```python
from build123d import *

# Parameters (mm, degrees)
SKETCH1_R            = 41.275
BODY_DEPTH           = 17.78
SKETCH2_R            = 41.275
SKETCH2_R_2          = 32.385
BOTTOM_INITIAL_DEPTH = 12.7
SKETCH3_R            = 32.385
SKETCH3_R_2          = 13.97
BOTTOM_STEM_DEPTH    = 7.62
SKETCH4_W            = 2.286
SKETCH4_H            = 2.54
SKETCH5_W            = 2.286
SKETCH5_H            = 2.54
CHAMFER1_SIZE        = 2.54
CHAMFER1_SIZE2       = 13.97
CUT_EXTRUDE3_REACH   = 63.02
SKETCH9_R            = 2.413
CIRPATTERN1_COUNT    = 6


with BuildPart() as part:
    # Sketch1 → Body (new body)
    with BuildSketch(Plane(origin=(0, 0, 0), x_dir=(1, 0, 0), z_dir=(0, 1, 0))):
        with Locations(Location((0, 0, 0), (0, 0, 270))):
            Circle(SKETCH1_R)
    extrude(amount=BODY_DEPTH)

    # Sketch2 → Bottom Initial (cut)
    with BuildSketch(Plane.XZ):
        with Locations(Location((0, 0, 0), (0, 0, 270))):
            Circle(SKETCH2_R)
        with Locations(Location((0, 0, 0), (0, 0, 270))):
            Circle(SKETCH2_R_2, mode=Mode.SUBTRACT)
    extrude(amount=-BOTTOM_INITIAL_DEPTH, mode=Mode.SUBTRACT)

    # Sketch3 → Bottom Stem (cut)
    with BuildSketch(Plane.XZ):
        with Locations(Location((0, 0, 0), (0, 0, 270))):
            Circle(SKETCH3_R)
        with Locations(Location((0, 0, 0), (0, 0, 270))):
            Circle(SKETCH3_R_2, mode=Mode.SUBTRACT)
    extrude(amount=-BOTTOM_STEM_DEPTH, mode=Mode.SUBTRACT)

    # Sketch4 → Top O ring (revolve, cut)
    with BuildSketch(Plane.XY, mode=Mode.PRIVATE) as top_o_ring_sk:
        with Locations((31.242, 10.16)):
            Rectangle(SKETCH4_W, SKETCH4_H)
    revolve(top_o_ring_sk.sketch.rotate(Axis((0, 18.669, 0), (0, -1, 0)), 270), axis=Axis((0, 18.669, 0), (0, -1, 0)), mode=Mode.SUBTRACT)

    # Sketch5 → Bottom O ring (revolve, cut)
    with BuildSketch(Plane.XY, mode=Mode.PRIVATE) as bottom_o_ring_sk:
        with Locations((12.827, 5.08)):
            Rectangle(SKETCH5_W, SKETCH5_H)
    revolve(bottom_o_ring_sk.sketch.rotate(Axis((0, 18.669, 0), (0, -1, 0)), 270), axis=Axis((0, 18.669, 0), (0, -1, 0)), mode=Mode.SUBTRACT)

    # Chamfer1
    chamfer1_edges = [part.edges().sort_by_distance(p)[0] for p in [
        (0, 0, 13.97),
    ]]
    chamfer1_side = [part.faces().sort_by_distance(p)[0] for p in [
        (0, 1.905, 13.97),
    ]]
    chamfer(chamfer1_edges, length=CHAMFER1_SIZE, length2=CHAMFER1_SIZE2, reference=chamfer1_side[0])

    # Sketch9 → Cut-Extrude3 (cut, up to next)
    with BuildSketch(Plane(origin=(0, 17.78, 0), x_dir=(1, 0, 0), z_dir=(0, 1, 0)), mode=Mode.PRIVATE) as cut_extrude3_sk1:
        with Locations(Location((-36.83, 0, 0), (0, 0, 270))):
            Circle(SKETCH9_R)
    cut_extrude3_tool1 = extrude(cut_extrude3_sk1.sketch, amount=-CUT_EXTRUDE3_REACH, mode=Mode.PRIVATE) & part.part
    cut_extrude3 = cut_extrude3_tool1.solids().sort_by_distance((-36.83, 17.78, 0))[0]
    add(cut_extrude3, mode=Mode.SUBTRACT)

    # CirPattern1: Cut-Extrude3 ×6 about axis
    cirpattern1_axis = Axis((0, 0, 0), (0, 1, 0))
    for i in range(1, CIRPATTERN1_COUNT):
        add(cut_extrude3.rotate(cirpattern1_axis, i * 360 / CIRPATTERN1_COUNT), mode=Mode.SUBTRACT)


solid = part.part
```
The listing builds one solid part. Answer for the finished solid, in the listing's coordinates (mm). A direction names the side the tool comes from. Give positions to 0.01 mm unless a question says otherwise; leave off trailing zeros. Order: outer loops, then holes, each group sorted by start corner. A loop starts at its lowest first (then second) coordinate and runs counter-clockwise, first axis right, second up. Notation, with made-up numbers: (-14, 59) -> (20, 59) arc R17 cw to (20, 84) -> close; hole circle Ø9 at (55.5, 69.5). An arc over 180 degrees is marked (long way). Answer as CSV lines item,"result". Start each with the question number.
Q1. A cutting plane is placed at B-B (y = 14). Determine the outline of the cut face in (x, z) (3 decimals).
Q2. Find the intervals of material crossed by L1, parallel to X at y = 15, z = 0 (3 decimals); L2, parallel to Y at x = 13.5, z = 23.5; L3, parallel to Y at x = 8.5, z = 11, in increasing order.
Q3. Determine the mould class of faces 1 (the cylindrical face through (-18.31, 10.18, 23.89)), 2 (the cylindrical face through (-17.491, 15.276, -34.125)), 3 (the flat face through (-10.3, 6.35, 6.1)) for opening direction X: pulls with the +X half, pulls with the -X half, needs draft (parallel to the pull), parting line crosses it, or undercut.
Q4. Given pin 1 (1.5 mm diameter, centred on x = 2, y = 11.5, fed in from -Z); pin 2 (5.5 mm diameter, centred on x = -18.42, z = 31.9, fed in from -Y); pin 3 (5 mm diameter, centred on y = 11.5, z = 5, fed in from -X); pin 4 (7.5 mm diameter, centred on x = 18.41, z = 31.9, fed in from +Y), each flat-ended and moving along its own axis, determine where each tip first touches the part or whether it passes through.
Q5. A cutting plane is placed at A-A (x = -36.83). Determine the outline of the cut face in (y, z), then the cut area to 3 significant figures.
Q6. Which of the six approach directions +Z, -Z, +X, -X, +Y, -Y give full straight-line access (tool end or side, diameter ignored) to faces 4 (the flat face through (-7, 7.62, -14)), 5 (the cylindrical face through (19.14, 15.276, 34.197)), 6 (the flat face through (-29, 8.89, 9))?
Results found:
1,outline,"circle Ø82.55 at (0, 0); hole circle Ø4.826 at (-36.83, 0); hole circle Ø4.826 at (-18.415, -31.896); hole circle Ø4.826 at (-18.415, 31.896); hole circle Ø4.826 at (18.415, -31.896); hole circle Ø4.826 at (18.415, 31.896); hole circle Ø4.826 at (36.83, 0)"
2,L1,"-41.275 to -39.243, -34.417 to 34.417, 39.243 to 41.275"
2,L2,"7.62 to 17.78"
2,L3,"2.53 to 3.81, 6.35 to 17.78"
3,face 1,"parting line crosses it"
3,face 2,"undercut"
3,face 3,"needs draft"
4,pin 1,"z = -32.36"
4,pin 2,"y = 12.7"
4,pin 3,"x = -41.18"
4,pin 4,"y = 17.78"
5,outline,"(12.7, -18.63) -> (17.78, -18.63) -> (17.78, -2.41) -> (12.7, -2.41) -> close; (12.7, 2.41) -> (17.78, 2.41) -> (17.78, 18.63) -> (12.7, 18.63) -> close"
5,area,"165 mm2"
6,face 4,"-Y"
6,face 5,"+Y, -Y"
6,face 6,"none"
